```python
from build123d import *

# Parameters (mm, degrees)
F1_DEPTH = 50.8
F2_R     = 6.35
F4_D     = 6.35
F6_DEPTH = 76.201


with BuildPart() as f1:
    # F0 (on Front) → F1 (new body, symmetric)
    with BuildSketch(Plane.XZ):
        with BuildLine():
            ThreePointArc((6.35, 44.45), (4.490128, 48.940128), (0, 50.8))
            Line((0, 50.8), (0, 0))
            Line((0, 0), (76.2, 0))
            ThreePointArc((76.2, 0), (74.340128, 4.490128), (69.85, 6.35))
            Line((69.85, 6.35), (6.35, 6.35))
            Line((6.35, 6.35), (6.35, 44.45))
        make_face()
    extrude(amount=F1_DEPTH, both=True)

    # F2
    f2_edges = [f1.edges().sort_by_distance(p)[0] for p in [
        (6.35, 0, 6.35),
    ]]
    fillet(f2_edges, radius=F2_R)

    # F4 (through all)
    with Locations(Plane(origin=(0, 0, 0), x_dir=(1, 0, 0), z_dir=(0, 0, -1))):
        with Locations((44.45, 25.979519), (44.45, -24.820481)):
            Hole(F4_D / 2)

    # F5 (on face) → F6 (cut, through all)
    with BuildSketch(Plane(origin=(0, 0, 0), x_dir=(0, -1, 0), z_dir=(-1, 0, 0))):
        with BuildLine():
            Line((-6.35, 34.426071), (-31.75, 34.426071))
            ThreePointArc((-31.75, 34.426071), (-38.1, 28.076071), (-31.75, 21.726071))
            Line((-31.75, 21.726071), (-6.35, 21.726071))
            ThreePointArc((-6.35, 21.726071), (0, 28.076071), (-6.35, 34.426071))
        make_face()
    extrude(amount=-F6_DEPTH, mode=Mode.SUBTRACT)


solid = f1.part
```
Part model, mm, in its own coordinate system. A direction names the side the tool comes from. Round coordinates to 2 decimals unless told otherwise and drop trailing zeros. Loops run counter-clockwise (first coordinate to the right, second up) from the corner with the lowest first, then second, coordinate; pieces in that order, holes last.
1. 3-axis set-ups, long thin cutter, end or side, ignore diameter. For faces 1 (the face through (41.52, -24.76, 3.22)), 2 (the face through (6.35, -1, 28)), 3 (the face through (3, 0, 28)): which of +Z, -Z, +X, -X, +Y, -Y reach the whole face in a straight line?
Solutions:
face 1: +Z, -Z
face 2: +Z, +X, +Y, -Y
face 3: +X, -X
2. Two-plate mould, pull along Z, no slides. Class faces 4 (the face through (4.54, -0.71, 48.89)), 5 (the face through (24, 50.8, 5)), 6 (the face through (3, 19, 34.426)): pulls with the +Z half, pulls with the -Z half, needs draft (parallel to the pull), parting line crosses it, or undercut.
Solutions:
face 4: pulls with the +Z half
face 5: needs draft
face 6: undercut
3. Drill centre lines: line 1 along Y through (x, z) = (44, 3); line 2 along X through (y, z) = (2, 42). Where is each one in solid material? Low to high.
Solutions:
line 1: y = -50.8 to -29.12, -22.84 to 21.68, 27.96 to 50.8
line 2: x = 0 to 6.35
4. Flat gauge pins, fed straight in: pin 1 (10 mm diameter, centred on x = 44.45, y = 24.82, fed in from -Z); pin 2 (1 mm diameter, centred on y = 40, z = 14.5, fed in from +X). Where does each tip first touch, or does it go through?
Solutions:
pin 1: stops at z = 0
pin 2: stops at x = 6.35
5. Slice it at B-B (y = 30). Give the cut face in (x, z).
Solutions:
outline: (0, 0) - (76.2, 0) arc R6.35 ccw to (69.85, 6.35) - (12.7, 6.35) arc R6.35 cw to (6.35, 12.7) - (6.35, 21.73) - (0, 21.73) - close; (0, 34.43) - (6.35, 34.43) - (6.35, 44.45) arc R6.35 ccw to (0, 50.8) - close
6. Slice it at C-C (z = 42). Give the cut face in (x, y).
Solutions:
outline: (0, -50.8) - (6.35, -50.8) - (6.35, 50.8) - (0, 50.8) - close
7. Slice it at A-A (x = 44.45). Give the cut face in (y, z).
Solutions:
outline: (-50.8, 0) - (-29.15, 0) - (-29.15, 6.35) - (-50.8, 6.35) - close; (-22.8, 0) - (21.65, 0) - (21.65, 6.35) - (-22.8, 6.35) - close; (28, 0) - (50.8, 0) - (50.8, 6.35) - (28, 6.35) - close
8. Slice it at D-D (y = -11.5). Give the cut face in (x, z).
Solutions:
outline: (0, 0) - (76.2, 0) arc R6.35 ccw to (69.85, 6.35) - (12.7, 6.35) arc R6.35 cw to (6.35, 12.7) - (6.35, 44.45) arc R6.35 ccw to (0, 50.8) - close
